Check sheet for the drawn part. Datum: minimum x, y, z corner. Units: mm. A direction names the side the tool comes from. Give positions to 0.01 mm unless a question says otherwise; leave off trailing zeros. Write each loop counter-clockwise with the first axis right and the second up, starting at its lowest first coordinate (ties: lowest second). Pieces come first, ordered by that corner, then holes. Notation, with made-up numbers: (72, -37.75) -> (90, -37.75) arc R29 cw to (90, -7.75) -> close; hole circle Ø5 at (34, 33.25). An arc over 180 degrees is marked (long way). Use CSV: the item, a comma, the result in double quotes. Start each with the question number.
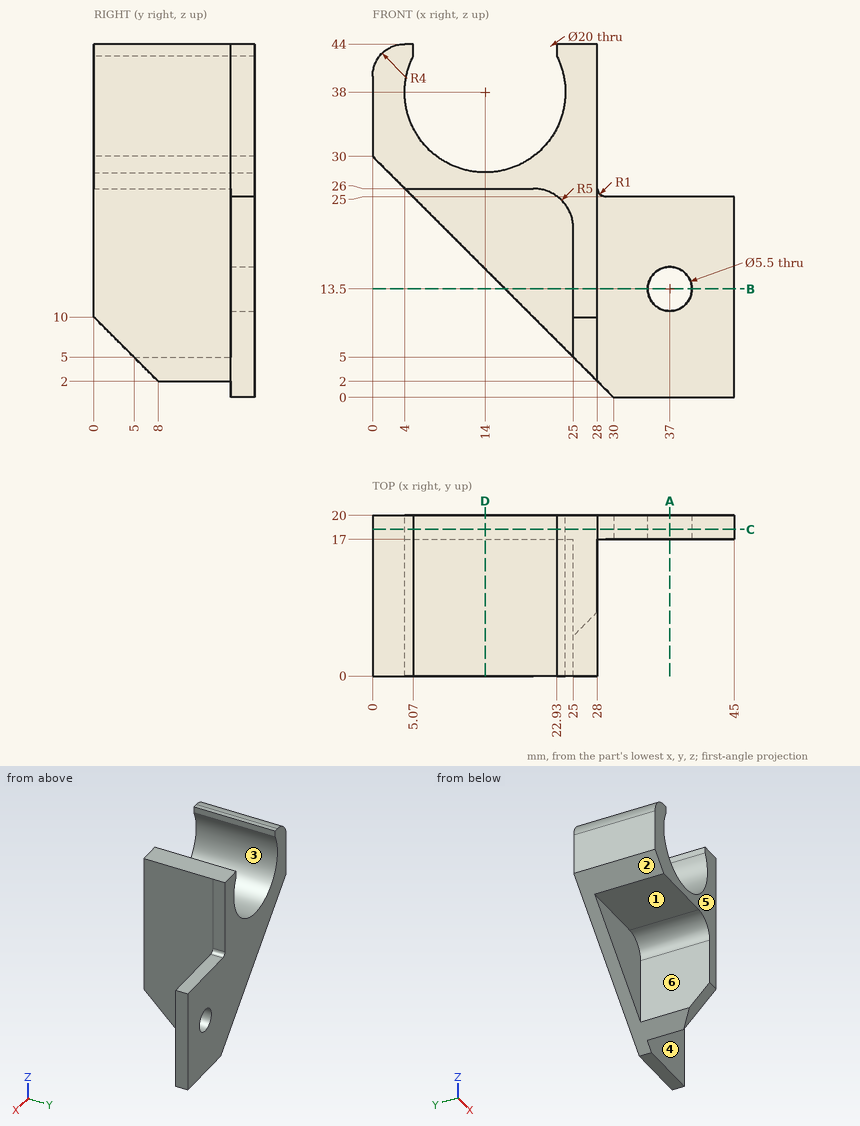
(1) Set-up check for the marked faces 4, 5 and 6: record each of +Z, -Z, +X, -X, +Y, -Y from which the full face is reachable in a straight line by a thin tool's end or side.
(2) Section check D-D on x = 14. Record the cut outline in (y, z).
(3) Section check B-B on z = 13.5. Record the cut outline in (x, y).
(4) Go/stop test with flat-tipped pins: pin 1 (4 mm diameter, centred on x = 14, y = 9.5, fed in from +Z); pin 2 (1.2 mm diameter, centred on y = 13.5, z = 43, fed in from +X); pin 3 (12 mm diameter, centred on y = 16.5, z = 8, fed in from -X). Record where each tip stops, or that it passes through.
(5) Thickness scan on line 1 (X direction, y = 4.5, z = 38); line 2 (Z direction, x = 37, y = 19.4); line 3 (Z direction, x = 14, y = 8.5). Record the ranges inside material, lowest first. Write a range as from..to.
(6) Draft check along X on the marked faces 1, 2 and 3. Enter one of: released by +X, released by -X, zero draft, split by the parting line, or undercut.
(7) Section check C-C on y = 18.25. Record the cut outline in (x, z), then the cut area to 3 significant figures.
(8) Section check A-A on x = 37. Record the cut outline in (y, z), then the cut area to 3 significant figures.
Data:
1,face 4,"+Z, -Z, +X, -Y"
1,face 5,"+Z, -Z, +X, -X, -Y"
1,face 6,"-Z, -X, -Y"
2,outline,"(0, 26) -> (17, 26) -> (17, 16) -> (20, 16) -> (20, 28) -> (0, 28) -> close"
3,outline,"(16.5, 17) -> (25, 17) -> (25, 0) -> (28, 0) -> (28, 17) -> (34.25, 17) -> (34.25, 20) -> (16.5, 20) -> close; (39.75, 17) -> (45, 17) -> (45, 20) -> (39.75, 20) -> close"
4,pin 1,"stops at z = 28.2"
4,pin 2,"stops at x = 28"
4,pin 3,"stops at x = 16.02"
5,line 1,"x = 0..4, 24..28"
5,line 2,"z = 0..10.75, 16.25..25"
5,line 3,"z = 26..28"
6,face 1,"zero draft"
6,face 2,"released by -X"
6,face 3,"undercut"
7,outline,"(0, 30) -> (30, 0) -> (45, 0) -> (45, 25) -> (29, 25) arc R1 cw to (28, 26) -> (28, 44) -> (22.93, 44) -> (22.93, 42.5) arc R10 cw (long way) to (5.07, 42.5) -> (5.07, 44) -> (4, 44) arc R4 ccw to (0, 40) -> close; hole circle Ø5.5 at (37, 13.5)"
7,area,"909 mm2"
8,outline,"(17, 0) -> (20, 0) -> (20, 10.75) -> (17, 10.75) -> close; (17, 16.25) -> (20, 16.25) -> (20, 25) -> (17, 25) -> close"
8,area,"58.5 mm2"
